```python
from build123d import *

# Parameters (mm, degrees)
F0_R      = 11
F0_W      = 87
F0_H      = 40
F0_R_2    = 3.75
F0_R_3    = 3
F0_R_4    = 2.25
F1_DEPTH  = 12
F2_R      = 3.75
F2_R_2    = 3
F2_R_3    = 2.25
F3_DEPTH  = 4.5
F4_R      = 20
F5_DEPTH  = 0.5
F6_R      = 16.5
F7_DEPTH  = 1.5
F8_R      = 16
F9_DEPTH  = 9
F10_R     = 13
F11_DEPTH = 10.5
F12_SIZE2 = 0.5
F12_SIZE  = 0.5
F13_SIZE2 = 0.49999
F13_SIZE  = 0.49999
F14_SIZE2 = 0.99999
F14_SIZE  = 0.99999


# Not quite as in the source:
# - a fillet or chamfer is up to 0.001 mm smaller than in the source, because OpenCascade refuses the exact size


with BuildPart() as f1:
    # F0 (on Front) → F1 (new body)
    with BuildSketch(Plane.XZ):
        with BuildLine():
            Line((-43.5, 20), (43.5, 20))
            Line((43.5, 20), (20.7387457553, 59.0790903836))
            ThreePointArc((20.7387457553, 59.0790903836), (0, 71), (-20.7387457553, 59.0790903836))
            Line((-20.7387457553, 59.0790903836), (-43.5, 20))
        make_face()
        with Locations((0, 47)):
            Circle(F0_R, mode=Mode.SUBTRACT)
        Rectangle(F0_W, F0_H)
        with Locations((-31.5, -15)):
            Circle(F0_R_2, mode=Mode.SUBTRACT)
        with Locations((-35.5, 14)):
            Circle(F0_R_2, mode=Mode.SUBTRACT)
        with Locations((31.5, -15)):
            Circle(F0_R_2, mode=Mode.SUBTRACT)
        with Locations((35.5, 14)):
            Circle(F0_R_2, mode=Mode.SUBTRACT)
        with Locations((-35.5, 14)):
            Circle(F0_R_2)
        with Locations((-35.5, 14)):
            Circle(F0_R_3, mode=Mode.SUBTRACT)
        with Locations((-31.5, -15)):
            Circle(F0_R_2)
        with Locations((-31.5, -15)):
            Circle(F0_R_4, mode=Mode.SUBTRACT)
        with Locations((35.5, 14)):
            Circle(F0_R_2)
        with Locations((35.5, 14)):
            Circle(F0_R_3, mode=Mode.SUBTRACT)
        with Locations((31.5, -15)):
            Circle(F0_R_2)
        with Locations((31.5, -15)):
            Circle(F0_R_4, mode=Mode.SUBTRACT)
    extrude(amount=F1_DEPTH)

    # F2 (on face) → F3 (cut)
    with BuildSketch(Plane.XZ.offset(12)):
        with Locations((-35.5, 14)):
            Circle(F2_R)
        with Locations((-35.5, 14)):
            Circle(F2_R_2, mode=Mode.SUBTRACT)
        with Locations((35.5, 14)):
            Circle(F2_R)
        with Locations((35.5, 14)):
            Circle(F2_R_2, mode=Mode.SUBTRACT)
        with Locations((-31.5, -15)):
            Circle(F2_R)
        with Locations((-31.5, -15)):
            Circle(F2_R_3, mode=Mode.SUBTRACT)
        with Locations((31.5, -15)):
            Circle(F2_R)
        with Locations((31.5, -15)):
            Circle(F2_R_3, mode=Mode.SUBTRACT)
    extrude(amount=-F3_DEPTH, mode=Mode.SUBTRACT)

    # F4 (on face) → F5 (cut)
    with BuildSketch(Plane(origin=(0, 0, 0), x_dir=(-1, 0, 0), z_dir=(0, 1, 0))):
        with Locations((0, 47)):
            Circle(F4_R)
    extrude(amount=-F5_DEPTH, mode=Mode.SUBTRACT)

    # F6 (on face) → F7 (cut)
    with BuildSketch(Plane(origin=(0, 0, 0), x_dir=(-1, 0, 0), z_dir=(0, 1, 0))):
        with Locations((0, 47)):
            Circle(F6_R)
    extrude(amount=-F7_DEPTH, mode=Mode.SUBTRACT)

    # F8 (on face) → F9 (cut)
    with BuildSketch(Plane(origin=(0, 0, 0), x_dir=(-1, 0, 0), z_dir=(0, 1, 0))):
        with Locations((0, 47)):
            Circle(F8_R)
    extrude(amount=-F9_DEPTH, mode=Mode.SUBTRACT)

    # F10 (on face) → F11 (cut)
    with BuildSketch(Plane(origin=(0, 0, 0), x_dir=(-1, 0, 0), z_dir=(0, 1, 0))):
        with Locations((0, 47)):
            Circle(F10_R)
    extrude(amount=-F11_DEPTH, mode=Mode.SUBTRACT)

    # F12
    f12_edges = [f1.edges().sort_by_distance(p)[0] for p in [
        (-32.119373, -12, 39.539545),
        (0, -12, 71),
        (-43.5, -12, 0),
        (32.119373, -12, 39.539545),
        (0, -12, -20),
        (43.5, -12, 0),
        (-35.25, -12, -15),
        (-39.25, -12, 14),
        (27.75, -12, -15),
        (31.75, -12, 14),
        (-11, -12, 47),
    ]]
    chamfer(f12_edges, length=F12_SIZE, length2=F12_SIZE2)

    # F13 (size 0.5 and 0.5 in the source; OpenCascade refuses exactly that, so slightly less here)
    f13_edges = [f1.edges().sort_by_distance(p)[0] for p in [
        (-32.119373, 0, 39.539545),
        (0, 0, 71),
        (-43.5, 0, 0),
        (32.119373, 0, 39.539545),
        (0, 0, -20),
        (43.5, 0, 0),
        (-33.75, 0, -15),
        (-38.5, 0, 14),
        (29.25, 0, -15),
        (32.5, 0, 14),
        (20, 0, 47),
    ]]
    chamfer(f13_edges, length=F13_SIZE, length2=F13_SIZE2)

    # F14 (size 1 and 1 in the source; OpenCascade refuses exactly that, so slightly less here)
    f14_edges = [f1.edges().sort_by_distance(p)[0] for p in [
        (16.5, -0.5, 47),
    ]]
    chamfer(f14_edges, length=F14_SIZE, length2=F14_SIZE2)


solid = f1.part
```
Read the model definition and answer for the solid it produces. Units are mm, in the model's axes. A direction names the side the tool comes from. Coordinates: 2 decimals unless noted, no trailing zeros. Loops run counter-clockwise (first coordinate to the right, second up) from the corner with the lowest first, then second, coordinate; pieces in that order, holes last. Notation, with made-up numbers: (15, 10.25) -> (51, 10.25) arc R8 cw to (51, 19.25) -> close; hole circle Ø9 at (82.5, -30). An arc over 180 degrees is marked (long way). Return JSON: item names as keys, results as strings.
Item 1: Flat-ended cylindrical pins translate along their axes: P1, Ø13, axis at x = 3, z = 46.5, coming from the +Y side; P2, Ø10, axis at x = -3.5, z = 39.5, coming from the +Y side; P3, Ø4, axis at y = -10.5, z = 46.5, coming from the -X side; P4, Ø4, axis at x = -32, y = -8, coming from the +Z side. Find the tip coordinate at first contact, or state that the pin passes through.
Answers:
{"P1": "passes through", "P2": "stops at y = -9", "P3": "stops at x = -29.23", "P4": "stops at z = 43.18"}
Item 2: Find section B-B (y = -5). Determine the outline of the cut face in (x, z), plus the area to 3 significant figures.
Answers:
{"outline": "(-43.5, -20) -> (43.5, -20) -> (43.5, 20) -> (20.74, 59.08) arc R24 ccw to (-20.74, 59.08) -> (-43.5, 20) -> close; hole circle Ø6 at (-35.5, 14); hole circle Ø4.5 at (-31.5, -15); hole circle Ø32 at (0, 47); hole circle Ø4.5 at (31.5, -15); hole circle Ø6 at (35.5, 14)", "area": "5,450 mm2"}
Item 3: Find the intervals of material crossed by probe 1 along Z at (x, y) = (-35.5, -8.4); probe 2 along Y at (x, z) = (-28, -15); probe 3 along Z at (x, y) = (-31.5, -8.4), in increasing order.
Answers:
{"probe 1": "z = -20 to 10.25, 17.75 to 33.74", "probe 2": "y = -7.5 to 0", "probe 3": "z = -20 to -18.75, -11.25 to 40.6"}
Item 4: For a pull along X with two mould halves and no side action, classify faces 4 (the conical face through (0.345, -0.135, 70.633)), 5 (the flat face through (43.5, -6, 0)), 6 (the flat face through (-37, -7.5, 17)) as +X half, -X half, draft (parallel to the pull), parting line (faces both ways), or undercut.
Answers:
{"face 4": "parting line", "face 5": "+X half", "face 6": "undercut"}
Item 5: For faces 1 (the flat face through (-31.74, -11.75, 39.69)), 2 (the flat face through (16, -1.5, 50)), 3 (the flat face through (34, -7.5, 17)), determine the directions among +Z, -Z, +X, -X, +Y, -Y from which every point of the face is accessible in a straight line to the end or side of a thin tool.
Answers:
{"face 1": "+Z, -X, -Y", "face 2": "+Y", "face 3": "-Y"}
Item 6: Find section D-D (x = 24.5). Determine the outline of the cut face in (y, z), plus the area to 3 significant figures.
Answers:
{"outline": "(-12, -19.5) -> (-11.5, -20) -> (-0.5, -20) -> (0, -19.5) -> (0, 51.63) -> (-0.5, 52.62) -> (-11.5, 52.62) -> (-12, 51.63) -> close", "area": "871 mm2"}
